```python
from build123d import *

# Parameters (mm, degrees)
CROQUIS1_R              = 3.75
CROQUIS1_W              = 3
CROQUIS1_H              = 12.3
SALIENTE_EXTRUIR1_DEPTH = 3


with BuildPart() as part:
    # Croquis1 → Saliente-Extruir1 (new body)
    with BuildSketch(Plane.XY):
        Polygon((94.108737778, 114.11492022), (26.558756283, 75.11492022), (26.558756283, -2.88507978), (94.108737778, -41.88507978), (161.658719273, -2.88507978), (161.658719273, 75.11492022), align=None)
        with Locations((37.817086532, 64.86492022)):
            Circle(CROQUIS1_R, mode=Mode.SUBTRACT)
        Polygon((101.681254795, 100.207027049), (100.19256624, 97.60242022), (110.844695242, 91.452410673), (112.333383798, 94.057017502), align=None, mode=Mode.SUBTRACT)
        Polygon((135.175742963, 80.868975289), (145.827871965, 74.718965742), (144.316560563, 72.12742022), (133.66443156, 78.277429767), align=None, mode=Mode.SUBTRACT)
        Polygon((133.66443156, -6.047589327), (135.175742963, -8.639134849), (145.827871965, -2.489125302), (144.316560563, 0.10242022), align=None, mode=Mode.SUBTRACT)
        Polygon((118.417179188, 90.544536596), (116.928490632, 87.939929767), (127.580619634, 81.78992022), (129.06930819, 84.394527049), align=None, mode=Mode.SUBTRACT)
        Polygon((129.06930819, -12.164686608), (118.417179188, -18.314696155), (116.928490632, -15.710089327), (127.580619634, -9.56007978), align=None, mode=Mode.SUBTRACT)
        Polygon((112.333383798, -21.827177061), (101.681254795, -27.977186608), (100.19256624, -25.37257978), (110.844695242, -19.222570233), align=None, mode=Mode.SUBTRACT)
        Polygon((77.372780314, -19.222570233), (75.884091759, -21.827177061), (86.536220761, -27.977186608), (88.024909317, -25.37257978), align=None, mode=Mode.SUBTRACT)
        Polygon((60.636855922, -9.56007978), (59.148167366, -12.164686608), (69.800296369, -18.314696155), (71.288984924, -15.710089327), align=None, mode=Mode.SUBTRACT)
        Polygon((43.900914994, 0.10242022), (54.553043996, -6.047589327), (53.041732593, -8.639134849), (42.389603591, -2.489125302), align=None, mode=Mode.SUBTRACT)
        Polygon((54.553043996, 78.277429767), (53.041732593, 80.868975289), (42.389603591, 74.718965742), (43.900914994, 72.12742022), align=None, mode=Mode.SUBTRACT)
        Polygon((59.148167366, 84.394527049), (69.800296369, 90.544536596), (71.288984924, 87.939929767), (60.636855922, 81.78992022), align=None, mode=Mode.SUBTRACT)
        Polygon((75.884091759, 94.057017502), (86.536220761, 100.207027049), (88.024909317, 97.60242022), (77.372780314, 91.452410673), align=None, mode=Mode.SUBTRACT)
        with Locations((151.900389024, 55.43992022)):
            Rectangle(CROQUIS1_W, CROQUIS1_H, mode=Mode.SUBTRACT)
        with Locations((151.900389024, 36.11492022)):
            Rectangle(CROQUIS1_W, CROQUIS1_H, mode=Mode.SUBTRACT)
        with Locations((151.900389024, 16.78992022)):
            Rectangle(CROQUIS1_W, CROQUIS1_H, mode=Mode.SUBTRACT)
    extrude(amount=SALIENTE_EXTRUIR1_DEPTH)


solid = part.part
```
Verification items for the finished model (mm, model axes). A direction names the side the tool comes from. Coordinates: 2 decimals unless noted, no trailing zeros. Loops run counter-clockwise (first coordinate to the right, second up) from the corner with the lowest first, then second, coordinate; pieces in that order, holes last. Notation, with made-up numbers: (70, 21) -> (74, 21) arc R23 cw to (74, 43) -> close; hole circle Ø5 at (69, 16.5). An arc over 180 degrees is marked (long way). Put each result on its own line as item: value.
1. Section check A-A, the plane y = 33. Record the boundary of the cut face in (x, z).
Result set:
outline: (26.56, 0) -> (150.4, 0) -> (150.4, 3) -> (26.56, 3) -> close; (153.4, 0) -> (161.66, 0) -> (161.66, 3) -> (153.4, 3) -> close
2. Gauge pin test, flat ends, axial feed: P1, Ø1.5, axis at x = 152, z = 1.5, coming from the +Y side; P2, Ø0.9, axis at x = 152.5, z = 2, coming from the +Y side. Record the tip position at first contact, or that the pin passes through.
Result set:
P1: stops at y = 81.12
P2: stops at y = 80.66
3. Section check B-B, the plane x = 37.5. Record the boundary of the cut face in (y, z).
Result set:
outline: (-9.2, 0) -> (61.13, 0) -> (61.13, 3) -> (-9.2, 3) -> close; (68.6, 0) -> (81.43, 0) -> (81.43, 3) -> (68.6, 3) -> close
4. Section check C-C, the plane z = 1.25. Give the number of separate pieces and of enclosed holes in the cut face, then the cut area to 3 significant figures.
Result set:
separate pieces: 1
enclosed holes: 16
area: 15,200 mm^2
5. Thickness scan on line 1 (X direction, y = 17.5, z = 2.35); line 2 (Y direction, x = 143, z = 0.5); line 3 (X direction, y = -24, z = 0.15). Record the ranges inside material, lowest first.
Result set:
line 1: x = 26.56 to 150.4, 153.4 to 161.66
line 2: y = -13.66 to -4.12, -0.66 to 72.89, 76.35 to 85.89
line 3: x = 63.13 to 79.65, 85.65 to 102.57, 108.57 to 125.09
6. Mould release check, pull along Y, two halves, no side actions. Record for faces 3 (the face through (61, 95, 1)), 4 (the face through (127.41, -22.66, 1.48)), 5 (the face through (140.427, -5.607, 1.479)), 6 (the face through (139.065, -2.93, 1.479)): pulls with the +Y half, pulls with the -Y half, needs draft (parallel to the pull), parting line crosses it, or undercut.
Result set:
face 3: pulls with the +Y half
face 4: pulls with the -Y half
face 5: undercut
face 6: undercut
7. Section check D-D, the plane y = 103.5. Record the boundary of the cut face in (x, z).
Result set:
outline: (75.72, 0) -> (112.49, 0) -> (112.49, 3) -> (75.72, 3) -> close
8. Tool access check on faces 1 (the face through (59.86, -22.11, 1.48)), 2 (the face through (105.444, -22.341, 1.479)). Record the directions out of +Z, -Z, +X, -X, +Y, -Y that give a thin tool (end or side, any length) a straight path to the whole face; none if there is none.
Result set:
face 1: +Z, -Z, -X, -Y
face 2: +Z, -Z
